from build123d import *

# Parameters (mm, degrees)
IZIM1_R                     = 13
IZIM1_R_2                   = 8
Y_KSEKLIK_EKSTR_ZYON2_DEPTH = 9
IZIM2_W                     = 60
IZIM2_H                     = 60
Y_KSEKLIK_EKSTR_ZYON3_DEPTH = 116
Y_KSEKLIK_EKSTR_ZYON4_DEPTH = 60
IZIM4_R                     = 20
KES_EKSTR_ZYON2_DEPTH       = 220
IZIM5_R                     = 12
KES_EKSTR_ZYON3_DEPTH       = 220
KES_EKSTR_ZYON4_DEPTH       = 220
Y_KSEKLIK_EKSTR_ZYON6_DEPTH = 20
Y_KSEKLIK_EKSTR_ZYON7_DEPTH = 20
Y_KSEKLIK_EKSTR_ZYON8_DEPTH = 20
IZIM12_W                    = 9.584184826
IZIM12_H                    = 42
KES_EKSTR_ZYON5_DEPTH       = 37
IZIM13_W                    = 27.999362569
IZIM13_H                    = 42
KES_EKSTR_ZYON6_DEPTH       = 9
Y_KSEKLIK_EKSTR_ZYON9_DEPTH = 44


with BuildPart() as part:
    # izim1 → Y_kseklik-Ekstr_zyon2 (new body)
    # profile 1 of 5: a face of its own
    with BuildSketch(Plane.XY):
        with Locations((14.305057501, -33.726417094)):
            Circle(IZIM1_R)
        with Locations((14.305057501, -33.726417094)):
            Circle(IZIM1_R_2, mode=Mode.SUBTRACT)
    # profile 2 of 5: a face of its own
    with BuildSketch(Plane.XY):
        with BuildLine():
            ThreePointArc((14.305057501, -20.726417094), (23.497445657, -24.534028939), (27.305057501, -33.726417094))
            Line((27.305057501, -33.726417094), (87.305057501, -33.726417094))
            ThreePointArc((87.305057501, -33.726417094), (91.112669346, -24.534028939), (100.305057501, -20.726417094))
            Line((100.305057501, -20.726417094), (100.305057501, 39.273582906))
            ThreePointArc((100.305057501, 39.273582906), (91.112669346, 43.08119475), (87.305057501, 52.273582906))
            Line((87.305057501, 52.273582906), (27.305057501, 52.273582906))
            ThreePointArc((27.305057501, 52.273582906), (23.497445657, 43.08119475), (14.305057501, 39.273582906))
            Line((14.305057501, 39.273582906), (14.305057501, -20.726417094))
        make_face()
    # profile 3 of 5: a face of its own
    with BuildSketch(Plane.XY):
        with Locations((100.305057501, -33.726417094)):
            Circle(IZIM1_R)
        with Locations((100.305057501, -33.726417094)):
            Circle(IZIM1_R_2, mode=Mode.SUBTRACT)
    # profile 4 of 5: a face of its own
    with BuildSketch(Plane.XY):
        with Locations((100.305057501, 52.273582906)):
            Circle(IZIM1_R)
        with Locations((100.305057501, 52.273582906)):
            Circle(IZIM1_R_2, mode=Mode.SUBTRACT)
    # profile 5 of 5: a face of its own
    with BuildSketch(Plane.XY):
        with Locations((14.305057501, 52.273582906)):
            Circle(IZIM1_R)
        with Locations((14.305057501, 52.273582906)):
            Circle(IZIM1_R_2, mode=Mode.SUBTRACT)
    extrude(amount=Y_KSEKLIK_EKSTR_ZYON2_DEPTH)

    # izim2 → Y_kseklik-Ekstr_zyon3 (add)
    with BuildSketch(Plane(origin=(0, 0, 0), x_dir=(-1, 0, 0), z_dir=(0, 0, -1))):
        with Locations((-57.305057501, 9.273582906)):
            Rectangle(IZIM2_W, IZIM2_H)
    extrude(amount=Y_KSEKLIK_EKSTR_ZYON3_DEPTH)

    # izim3 → Y_kseklik-Ekstr_zyon4 (add)
    with BuildSketch(Plane.XZ.offset(20.726417094)):
        with BuildLine():
            ThreePointArc((27.305057501, -116), (57.305057501, -146), (87.305057501, -116))
            Line((87.305057501, -116), (67.305057501, -116))
            ThreePointArc((67.305057501, -116), (57.305057501, -126), (47.305057501, -116))
            Line((47.305057501, -116), (27.305057501, -116))
        make_face()
    extrude(amount=-Y_KSEKLIK_EKSTR_ZYON4_DEPTH)

    # izim4 → Kes-Ekstr_zyon2 (cut)
    with BuildSketch(Plane.XZ.offset(20.726417094)):
        with Locations(Location((57.305057501, -116, 0), (0, 0, 270))):
            Circle(IZIM4_R)
    extrude(amount=-KES_EKSTR_ZYON2_DEPTH, mode=Mode.SUBTRACT)

    # izim5 → Kes-Ekstr_zyon3 (cut)
    with BuildSketch(Plane.XZ.offset(20.726417094)):
        with Locations(Location((57.305057501, -36, 0), (0, 0, 270))):
            Circle(IZIM5_R)
    extrude(amount=-KES_EKSTR_ZYON3_DEPTH, mode=Mode.SUBTRACT)

    # izim6 → Kes-Ekstr_zyon4 (cut)
    with BuildSketch(Plane(origin=(0, -20.726417094, 0), x_dir=(-1, 0, 0), z_dir=(0, -1, 0))):
        with BuildLine():
            ThreePointArc((-27.305057501, 116), (-36.091854066, 137.213203436), (-57.305057501, 146))
            Line((-57.305057501, 146), (-57.305057501, 136))
            ThreePointArc((-57.305057501, 136), (-43.162921878, 130.142135624), (-37.305057501, 116))
            ThreePointArc((-37.305057501, 116), (-43.162921878, 101.857864376), (-57.305057501, 96))
            Line((-57.305057501, 96), (-57.305057501, 48))
            ThreePointArc((-57.305057501, 48), (-48.819776127, 44.485281374), (-45.305057501, 36))
            Line((-45.305057501, 36), (-27.305057501, 36))
            Line((-27.305057501, 36), (-27.305057501, 116))
        make_face()
    extrude(amount=-KES_EKSTR_ZYON4_DEPTH, mode=Mode.SUBTRACT)



with BuildPart() as body_2:
    # izim7 → Y_kseklik-Ekstr_zyon6 (new body)
    with BuildSketch(Plane(origin=(0, -0.726417094, 0), x_dir=(-1, 0, 0), z_dir=(0, -1, 0))):
        with BuildLine():
            Line((-57.305057501, 131.175251222), (-57.305057501, 135.999344695))
            ThreePointArc((-57.305057501, 135.999344695), (-77.304402197, 116), (-57.305057501, 96.000655305))
            Line((-57.305057501, 96.000655305), (-57.305057501, 100.824748778))
            ThreePointArc((-57.305057501, 100.824748778), (-72.480308724, 116), (-57.305057501, 131.175251222))
        make_face()
    extrude(amount=-Y_KSEKLIK_EKSTR_ZYON6_DEPTH)


with BuildPart() as part_1:
    add(part.part)

    add(body_2.part)  # Y_kseklik-Ekstr_zyon7 merges body 2
    # izim10 → Y_kseklik-Ekstr_zyon7 (add)
    with BuildSketch(Plane(origin=(0, 19.273582906, 0), x_dir=(-1, 0, 0), z_dir=(0, -1, 0))):
        with BuildLine():
            Line((-57.305057501, 96), (-57.305057501, 107))
            ThreePointArc((-57.305057501, 107), (-66.305057501, 116), (-57.305057501, 125))
            Line((-57.305057501, 125), (-57.305057501, 136))
            ThreePointArc((-57.305057501, 136), (-77.305057501, 116), (-57.305057501, 96))
        make_face()
    extrude(amount=-Y_KSEKLIK_EKSTR_ZYON7_DEPTH)

    # izim11 → Y_kseklik-Ekstr_zyon8 (add)
    with BuildSketch(Plane(origin=(0, -0.726417094, 0), x_dir=(-1, 0, 0), z_dir=(0, -1, 0))):
        with BuildLine():
            Line((-57.305057501, 43), (-57.305057501, 48))
            ThreePointArc((-57.305057501, 48), (-65.790338876, 27.514718626), (-45.305057501, 36))
            Line((-45.305057501, 36), (-50.305057501, 36))
            ThreePointArc((-50.305057501, 36), (-62.25480497, 31.050252532), (-57.305057501, 43))
        make_face()
    extrude(amount=-Y_KSEKLIK_EKSTR_ZYON8_DEPTH)

    # izim12 → Kes-Ekstr_zyon5 (cut)
    with BuildSketch(Plane(origin=(0, 0, -36), x_dir=(-1, 0, 0), z_dir=(0, 0, -1))):
        with Locations((-32.097149914, 9.273582906)):
            Rectangle(IZIM12_W, IZIM12_H)
    extrude(amount=-KES_EKSTR_ZYON5_DEPTH, mode=Mode.SUBTRACT)

    # izim13 → Kes-Ekstr_zyon6 (cut)
    with BuildSketch(Plane.ZY.offset(-36.889242327)):
        with Locations((-12.999681285, 9.273582906)):
            Rectangle(IZIM13_W, IZIM13_H)
    extrude(amount=-KES_EKSTR_ZYON6_DEPTH, mode=Mode.SUBTRACT)

    # izim15 → Y_kseklik-Ekstr_zyon9 (add)
    with BuildSketch(Plane.XZ.offset(-30.273582906)):
        with BuildLine():
            Line((45.889242327, -26.999362569), (36.889242327, -36))
            ThreePointArc((36.889242327, -36), (36.888923612, -26.999681284), (45.889242327, -26.999362569))
        make_face()
    extrude(amount=Y_KSEKLIK_EKSTR_ZYON9_DEPTH)


solid = part_1.part
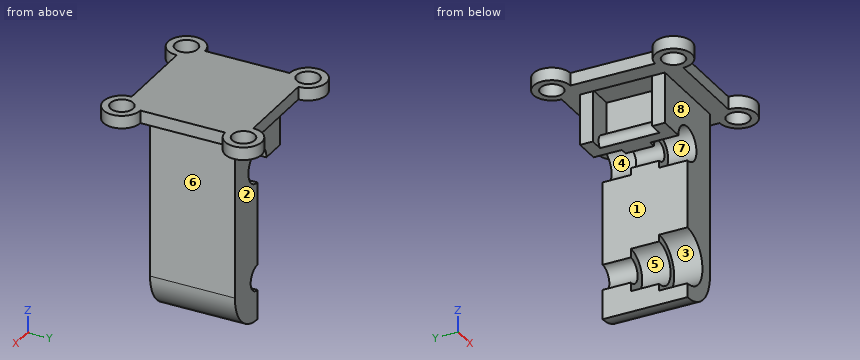
Geometry: final body of the model. Coordinates: model frame, mm. Face numbers are marked on the shaded views. A direction names the side the tool comes from. Give positions to 0.01 mm unless a question says otherwise; leave off trailing zeros. Order: outer loops, then holes, each group sorted by start corner. A loop starts at its lowest first (then second) coordinate and runs counter-clockwise, first axis right, second up. Notation, with made-up numbers: (-18, -5.75) - (28, -5.75) arc R26 ccw to (28, 18.25) - close; hole circle Ø10 at (83, 45). An arc over 180 degrees is marked (long way). Use CSV: the item, a comma, the result in double quotes.
1. Section query D-D (z = -94). Output: boundary loops of the cut face in (x, y).
Answers below:
outline,"(57.31, -20.73) - (87.31, -20.73) - (87.31, 39.27) - (57.31, 39.27) - close"
2. Section query C-C (x = 29.5). Output: boundary loops of the cut face in (y, z), plus the area to 3 significant figures.
Answers below:
outline,"(-33.73, 0) - (-20.73, 0) - (-20.73, -36) - (-11.73, -36) - (-11.73, 1) - (30.27, 1) - (30.27, -36) - (39.27, -36) - (39.27, 0) - (52.27, 0) - (52.27, 9) - (-33.73, 9) - close"
area,"1,380 mm2"
3. Material intervals for line 1 along Y through (x, z) = (37.5, -17.5); line 2 along Z through (x, y) = (60, -3.5); line 3 along Z through (x, y) = (32, 34.5), sorted ascending. Write a range as from..to.
Answers below:
line 1,"-20.73..-11.73, 30.27..39.27"
line 2,"-145.88..-135.82, -96.18..-47.69, -24.31..9"
line 3,"-36..9"
4. Access query for the marked faces 1, 2, 3, 4 and 5. Directions: +Z, -Z, +X, -X, +Y, -Y. A direction counts if a zero-diameter tool reaches every point of the face in a straight line with its end or side. Return the directions, or none.
Answers below:
face 1,"-Z, -X, +Y, -Y"
face 2,"-Z, +X, -X, +Y"
face 3,"none"
face 4,"+Y"
face 5,"-X, -Y"
5. Section query A-A (x = 10). Output: boundary loops of the cut face in (y, z), plus the area to 3 significant figures.
Answers below:
outline,"(-45.99, 0) - (-40.47, 0) - (-40.47, 9) - (-45.99, 9) - close; (-26.98, 0) - (-21.46, 0) - (-21.46, 9) - (-26.98, 9) - close; (40.01, 0) - (45.53, 0) - (45.53, 9) - (40.01, 9) - close; (59.02, 0) - (64.54, 0) - (64.54, 9) - (59.02, 9) - close"
area,"199 mm2"
6. Section query B-B (y = 37). Output: boundary loops of the cut face in (x, z).
Answers below:
outline,"(14.31, 0) - (27.31, 0) - (27.31, -36) - (45.31, -36) arc R12 cw (long way) to (57.31, -48) - (57.31, -107) arc R9 cw to (57.31, -125) - (57.31, -146) arc R30 ccw to (87.31, -116) - (87.31, 0) - (100.31, 0) - (100.31, 9) - (14.31, 9) - close"
7. Mould query, pull axis X, two halves, no side actions, for the marked faces 6, 7 and 8. Classes: +X half, -X half, draft (parallel to the pull), parting line (faces both ways), or undercut.
Answers below:
face 6,"+X half"
face 7,"undercut"
face 8,"draft"
8. Contact query for flat-ended pins moving along their axis: pin 1 (5 mm diameter, centred on y = -21, z = -125, fed in from +X); pin 2 (2.5 mm diameter, centred on y = -16, z = -11.5, fed in from -X); pin 3 (5 mm diameter, centred on y = 30, z = -100.5, fed in from +X). Output: stop coordinate, or through.
Answers below:
pin 1,"x = 86.59"
pin 2,"x = 27.31"
pin 3,"x = 87.31"
